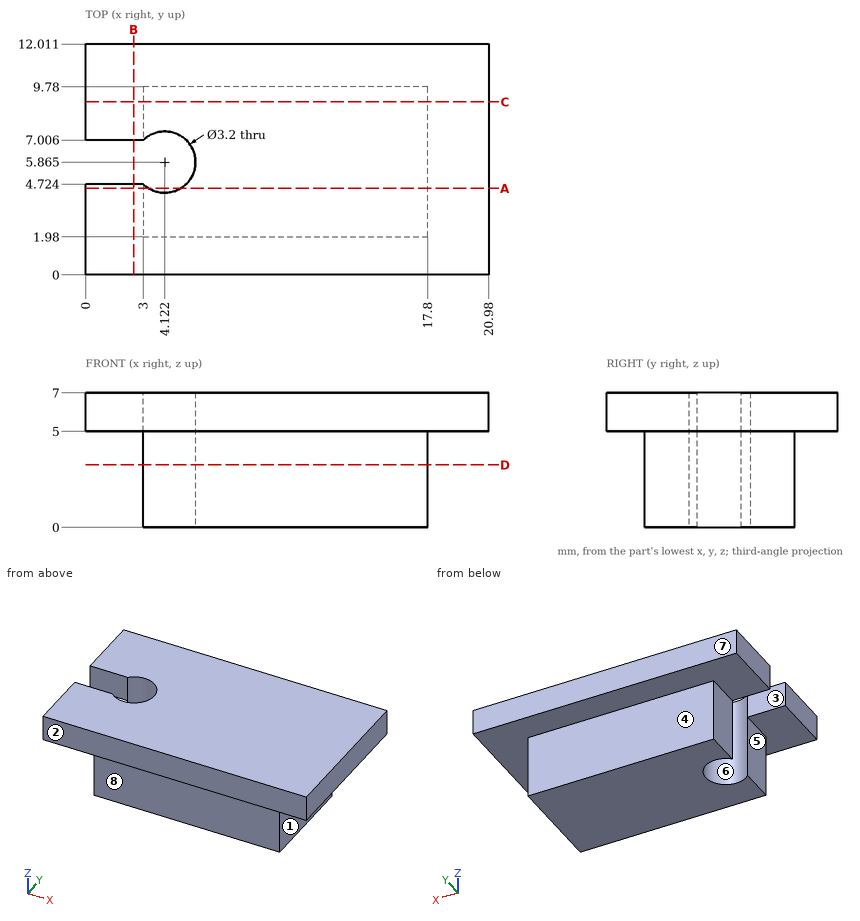
Study the drawing (mm; zero at the part's minimum x, y, z) and answer. A direction names the side the tool comes from. Coordinates: 2 decimals unless noted, no trailing zeros. Write each loop counter-clockwise with the first axis right and the second up, starting at its lowest first coordinate (ties: lowest second). Pieces come first, ordered by that corner, then holes. Notation, with made-up numbers: M 30.25,89.25 L 37.25,89.25 A23 cw 37.25,107.25 Z; hole C 14,39.25 d11. An arc over 180 degrees is marked long. Use one line per item in the form item = value.
Item 1: Given P1, Ø2, axis at y = 8, z = 3, coming from the -X side; P2, Ø1.5, axis at x = 7.5, z = 1.5, coming from the -Y side; P3, Ø2.5, axis at x = 14, z = 3.5, coming from the +Y side, each flat-ended and moving along its own axis, determine where each tip first touches the part or whether it passes through.
Model answer:
P1 = 3
P2 = 1.98
P3 = 9.78
Item 2: Find section A-A, the plane y = 4.5. Give the vertices of the cut face in (x, z), plus the area to 3 significant figures.
Model answer:
outline = M 0,5 L 3,5 L 3,0 L 3.29,0 L 3.29,7 L 0,7 Z; M 4.96,0 L 17.8,0 L 17.8,5 L 20.98,5 L 20.98,7 L 4.96,7 Z
area = 104 mm2
Item 3: Find section C-C, the plane y = 9. Give the vertices of the cut face in (x, z), plus the area to 3 significant figures.
Model answer:
outline = M 0,5 L 3,5 L 3,0 L 17.8,0 L 17.8,5 L 20.98,5 L 20.98,7 L 0,7 Z
area = 116 mm2
Item 4: Find section D-D, the plane z = 3.25. Give the vertices of the cut face in (x, y) (1 decimal), plus the area to 3 significant figures.
Model answer:
outline = M 3,2 L 17.8,2 L 17.8,9.8 L 3,9.8 L 3,7 A1.6 cw long 3,4.7 Z
area = 108 mm2
Item 5: For the marked faces 1, 2, 3, 4 and 5, determine the directions among +Z, -Z, +X, -X, +Y, -Y from which every point of the face is accessible in a straight line to the end or side of a thin tool.
Model answer:
face_1 = -Z, +X, +Y, -Y
face_2 = +Z, -Z, +X, -X, -Y
face_3 = +Z, -Z, -X
face_4 = -Z, +X, -X, +Y
face_5 = -Z, -X, +Y, -Y
Item 6: Find section B-B, the plane x = 2.5. Give the vertices of the cut face in (y, z).
Model answer:
outline = M 0,5 L 4.72,5 L 4.72,7 L 0,7 Z; M 7.01,5 L 12.01,5 L 12.01,7 L 7.01,7 Z
Item 7: The mould has two halves that part along Y. Classify the marked faces 6, 7 and 8: released by +Y, released by -Y, zero draft, split by the parting line, or undercut.
Model answer:
face_6 = undercut
face_7 = released by +Y
face_8 = released by -Y
Item 8: Find the intervals of material crossed by probe 1 along Y at (x, z) = (17.75, 1.25); probe 2 along X at (y, z) = (8.75, 1.75); probe 3 along Y at (x, z) = (4, 2.25), in increasing order.
Model answer:
probe_1 = 1.98 to 9.78
probe_2 = 3 to 17.8
probe_3 = 1.98 to 4.27, 7.46 to 9.78
